from build123d import *

# Parameters (mm, degrees)
F1_DEPTH = 75.8
F2_DEPTH = 48


with BuildPart() as f1:
    # F0 (on Front) → F1 (new body)
    with BuildSketch(Plane.XZ):
        Polygon((80, 90), (-80, 90), (-80, 70), (-10, 70), (-10, -70), (-75, -70), (-75, -90), (75, -90), (75, -70), (10, -70), (10, 70), (80, 70), align=None)
    extrude(amount=F1_DEPTH)

    # F0 (on Front) → F2 (join, symmetric)
    with BuildSketch(Plane.XZ):
        Polygon((80, 90), (-80, 90), (-80, 70), (-10, 70), (-10, -70), (-75, -70), (-75, -90), (75, -90), (75, -70), (10, -70), (10, 70), (80, 70), align=None)
    extrude(amount=F2_DEPTH, both=True)


solid = f1.part
Source: CAD feature listing. Evaluate the final solid. Frame: model axes, mm. A direction names the side the tool comes from. Give positions to 0.01 mm unless a question says otherwise; leave off trailing zeros. Write each loop counter-clockwise with the first axis right and the second up, starting at its lowest first coordinate (ties: lowest second). Pieces come first, ordered by that corner, then holes. Notation, with made-up numbers: M 4.5,61.5 L 43.5,61.5 A7 cw 43.5,67.5 Z; hole C 48.5,-33.75 d8. An arc over 180 degrees is marked long. Answer as a JSON object with one key per item and string values.
Q1. Ray query, line 1 along Z through (x, y) = (-12.5, 24); line 2 along X through (y, z) = (-21, 11); line 3 along X through (y, z) = (0.5, -78.5). Return the intervals inside material, ascending.
Geometry check:
{"line 1": "z = -90 to -70, 70 to 90", "line 2": "x = -10 to 10", "line 3": "x = -75 to 75"}
Q2. Cut plane C-C, the plane z = 52. Return the cut outline in (x, y), then the cut area to 3 significant figures.
Geometry check:
{"outline": "M -10,-75.8 L 10,-75.8 L 10,48 L -10,48 Z", "area": "2,480 mm^2"}
Q3. Cut plane A-A, the plane x = -23. Return the cut outline in (y, z), then the cut area to 3 significant figures.
Geometry check:
{"outline": "M -75.8,-90 L 48,-90 L 48,-70 L -75.8,-70 Z; M -75.8,70 L 48,70 L 48,90 L -75.8,90 Z", "area": "4,950 mm^2"}
Q4. Cut plane B-B, the plane y = -37. Return the cut outline in (x, z), then the cut area to 3 significant figures.
Geometry check:
{"outline": "M -80,70 L -10,70 L -10,-70 L -75,-70 L -75,-90 L 75,-90 L 75,-70 L 10,-70 L 10,70 L 80,70 L 80,90 L -80,90 Z", "area": "9,000 mm^2"}
Q5. Mould query, pull axis Z, two halves, no side actions, for faces 6 (the face through (10, -15, -1)), 7 (the face through (1, -15, 90)), 8 (the face through (75, -15, -80)), 9 (the face through (45, -15, 70)). Classes: +Z half, -Z half, draft (parallel to the pull), parting line (faces both ways), or undercut.
Geometry check:
{"face 6": "undercut", "face 7": "+Z half", "face 8": "draft", "face 9": "undercut"}
Q6. Contact query for flat-ended pins moving along their axis: P1, Ø10, axis at y = -31.5, z = -80, coming from the -X side; P2, Ø10, axis at y = -9, z = -23, coming from the +X side; P3, Ø10, axis at y = 5.5, z = -75.5, coming from the +X side. Output: stop coordinate, or through.
Geometry check:
{"P1": "stops at x = -75", "P2": "stops at x = 10", "P3": "stops at x = 75"}
Q7. Access query for faces 1 (the face through (-80, -15, 80)), 2 (the face through (-42, -15, -70)), 3 (the face through (43, -15, -70)), 4 (the face through (0, 48, 7)), 5 (the face through (-75, -15, -80)). Directions: +Z, -Z, +X, -X, +Y, -Y. A direction counts if a zero-diameter tool reaches every point of the face in a straight line with its end or side. Return the directions, or none.
Geometry check:
{"face 1": "+Z, -Z, -X, +Y, -Y", "face 2": "-X, +Y, -Y", "face 3": "+X, +Y, -Y", "face 4": "+Z, -Z, +X, -X, +Y", "face 5": "-Z, -X, +Y, -Y"}
